from build123d import *

# Parameters (mm, degrees)
F1_DEPTH = 400
F3_DEPTH = 500
F4_W     = 200
F4_H     = 199.3884497032
F5_DEPTH = 800


with BuildPart() as f1:
    # F0 (on Front) → F1 (new body)
    with BuildSketch(Plane.XZ):
        Polygon((400, 151.8551181662), (0, 151.8551181662), (0, 106.8551181662), (-260.0718909173, -42.6862191112), (-160.6825062296, -215.5373229158), (400, 106.8551181662), align=None)
    extrude(amount=F1_DEPTH)

    # F2 (on face) → F3 (cut, symmetric)
    with BuildSketch(Plane(origin=(-46.1750628055, 0, 80.3044570531), x_dir=(0.8669063031, 0, 0.4984711243), z_dir=(-0.4984711243, 0, 0.8669063031))):
        Polygon((75.6953914767, -400), (-246.735809115, -300), (-246.735809115, -400), align=None)
        Polygon((-246.735809115, 0), (-246.735809115, -100), (53.264190885, -6.956895161), (53.264190885, 0), align=None)
    extrude(amount=F3_DEPTH, both=True, mode=Mode.SUBTRACT)

    # F4 (on face) → F5 (join)
    with BuildSketch(Plane(origin=(-213.8968281118, 0, -122.9906761643), x_dir=(0, -1, 0), z_dir=(-0.8669063031, 0, -0.4984711243))):
        with Locations((200, -7.0608493994)):
            Rectangle(F4_W, F4_H)
    extrude(amount=F5_DEPTH)


solid = f1.part
Read the model definition and answer for the solid it produces. Units are mm, in the model's axes. A direction names the side the tool comes from. Give positions to 0.01 mm unless a question says otherwise; leave off trailing zeros. Loops run counter-clockwise (first coordinate to the right, second up) from the corner with the lowest first, then second, coordinate; pieces in that order, holes last. Notation, with made-up numbers: (-5.5, 75.25) -> (7.5, 75.25) arc R17 ccw to (7.5, 86.25) -> close; hole circle Ø10 at (-32.75, -27.75). An arc over 180 degrees is marked (long way). Use a Markdown table: item, result.
Q1. Each of these flat-tipped pins is pushed along its axis until it touches: pin 1 (13.5 mm diameter, centred on y = -180.5, z = 135.5, fed in from -X); pin 2 (2 mm diameter, centred on y = -54, z = 34, fed in from +X); pin 3 (5 mm diameter, centred on x = -772.5, y = -108, fed in from -Z). Where does it stop, or does it pass through?
Solved:
| item | result |
|---|---|
| pin 1 | stops at x = 0 |
| pin 2 | stops at x = 275.03 |
| pin 3 | stops at z = -568.77 |
Q2. Section C-C, the plane z = -154.5 is taken. Determine the outline of the cut face in (x, y), then the cut area to 3 significant figures.
Solved:
| item | result |
|---|---|
| outline | (-454.53, -300) -> (-195.78, -300) -> (-54.53, -337.98) -> (-54.53, -62.02) -> (-195.78, -100) -> (-454.53, -100) -> close |
| area | 85,400 mm^2 |
Q3. A tool of negligible diameter and unlimited length cuts with its end or side. For faces 1 (the face through (49, -3.53, 21.64)), 2 (the face through (0, -197, 130)), 3 (the face through (400, -197, 129)), from which of +Z, -Z, +X, -X, +Y, -Y can it reach the whole face along a straight path? Write none if from no direction.
Solved:
| item | result |
|---|---|
| face 1 | -Z, -X, +Y |
| face 2 | +Z, -X, +Y, -Y |
| face 3 | +Z, -Z, +X, +Y, -Y |
Q4. Section D-D, the plane x = -668 is taken. Determine the outline of the cut face in (y, z).
Solved:
| item | result |
|---|---|
| outline | (-300, -507.24) -> (-100, -507.24) -> (-100, -277.24) -> (-300, -277.24) -> close |
Q5. Find the intervals of material crossed by line 1 along Y through (x, z) = (-671, -360); line 2 along Y through (x, z) = (-91, -51); line 3 along X through (y, z) = (-191, -496), in increasing order.
Solved:
| item | result |
|---|---|
| line 1 | y = -300 to -100 |
| line 2 | y = -344.17 to -55.83 |
| line 3 | x = -922.24 to -648.44 |
Q6. Section A-A, the plane y = -142.5 is taken. Determine the outline of the cut face in (x, z).
Solved:
| item | result |
|---|---|
| outline | (-953.6, -441.46) -> (-854.21, -614.31) -> (400, 106.86) -> (400, 151.86) -> (0, 151.86) -> (0, 106.86) -> close |
Q7. Section B-B, the plane x = -243 is taken. Determine the outline of the cut face in (y, z).
Solved:
| item | result |
|---|---|
| outline | (-306.11, -32.87) -> (-300, -72.38) -> (-300, -262.87) -> (-100, -262.87) -> (-100, -72.38) -> (-93.89, -32.87) -> close |
